Can you work these out from the model? Positions are in its coordinate system, mm. A direction names the side the tool comes from. Coordinates: 2 decimals unless noted, no trailing zeros. Order: outer loops, then holes, each group sorted by start corner. A loop starts at its lowest first (then second) coordinate and runs counter-clockwise, first axis right, second up. Notation, with made-up numbers: (-6.5, 77) -> (1.5, 77) arc R7 ccw to (1.5, 85) -> close; hole circle Ø1 at (50.5, 83). An arc over 180 degrees is marked (long way). Answer as a JSON object with one key per item and string values. Group by question number.
(1) For pin 1 (1.5 mm diameter, centred on x = -2.5, z = 3.5, fed in from -Y); pin 2 (2 mm diameter, centred on y = -2, z = 5.5, fed in from -X), each with a flat end and sliding along its axis, tell me the tip position at first contact or that it passes through.
(2) I want a section at A-A, the plane x = 6. List the corners of the cut face in (y, z) for me.
(3) I need wall thicknesses on line 1 (Y direction, x = 1, z = 5.5); line 2 (Y direction, x = 6.5, z = 1.25); line 3 (Y direction, x = -10.25, z = 2.5). Which ranges of each line are inside material? Lowest first, please.
(4) If we mould it in two halves opening along Y, with no side actions, what happens to faces 6 (the cylindrical face through (-12.62, -1.44, 3.13)), 7 (the cylindrical face through (12.62, 1.44, 3.13)), 8 (the cylindrical face through (7.67, -8.13, 3.13))? For each: pulls with the +Y half, pulls with the -Y half, needs draft (parallel to the pull), parting line crosses it, or undercut.
(5) I want a section at B-B, the plane z = 3. State how many separate pieces and enclosed holes the cut face has, plus the area to 3 significant figures.
(6) I want a section at C-C, the plane y = -4. List the corners of the cut face in (x, z) for me.
(7) Which directions (+Z, -Z, +X, -X, +Y, -Y) give clear straight access to the entire face, cutting with the end or side of a thin tool? Please do faces 1 (the cylindrical face through (-9.66, -5.51, 3.13)), 2 (the cylindrical face through (-2.44, 8.54, 3.13)), 3 (the cylindrical face through (5.51, -9.66, 3.13)), 4 (the cylindrical face through (7.895, 4.048, 3.131)), 5 (the cylindrical face through (-5.51, 9.66, 3.13)).
from build123d import *

# Parameters (mm, degrees)
SKETCH3_R         = 12.7
GEARBODY_DEPTH    = 6.35
TOOTHCUT_DEPTH    = 20.05
CIRPATTERN1_COUNT = 12
BOREDIA_R         = 2.5
BOREDIA_R_2       = 1.27
BORE_DEPTH        = 12700


with BuildPart() as part:
    # Sketch3 → gearBody (new body)
    with BuildSketch(Plane.XY):
        Circle(SKETCH3_R)
    extrude(amount=GEARBODY_DEPTH)

    # Sketch2 → toothCut (cut, through all)
    with BuildSketch(Plane.XY):
        with BuildLine():
            ThreePointArc((8.504981128, -1.619352377), (8.564111751, -1.270037802), (8.608901587, -0.918596522))
            ThreePointArc((8.608901587, -0.918596522), (8.867488023, -0.436790342), (9.388953743, -0.272237485))
            ThreePointArc((9.388953743, -0.272237485), (11.599176183, 0.135890641), (13.30511426, 1.599252209))
            ThreePointArc((13.30511426, 1.599252209), (13.255912686, -1.96582094), (12.268366453, -5.391739765))
            ThreePointArc((12.268366453, -5.391739765), (11.060534793, -3.49627294), (9.063879737, -2.464274691))
            ThreePointArc((9.063879737, -2.464274691), (8.61261217, -2.155467755), (8.504981128, -1.619352377))
        make_face()
    toothcut = extrude(amount=TOOTHCUT_DEPTH, mode=Mode.SUBTRACT)

    # CirPattern1: toothCut ×12 about axis
    cirpattern1_axis = Axis((0, 0, 0), (0, 0, 1))
    for i in range(1, CIRPATTERN1_COUNT):
        add(toothcut.rotate(cirpattern1_axis, i * 360 / CIRPATTERN1_COUNT), mode=Mode.SUBTRACT)

    # boreDia → bore (cut, symmetric)
    with BuildSketch(Plane.XY):
        Circle(BOREDIA_R)
        with Locations((0, 6.35)):
            Circle(BOREDIA_R_2)
        with Locations((6.35, 0)):
            Circle(BOREDIA_R_2)
        with Locations((-6.35, 0)):
            Circle(BOREDIA_R_2)
        with Locations((0, -6.35)):
            Circle(BOREDIA_R_2)
    extrude(amount=BORE_DEPTH, both=True, mode=Mode.SUBTRACT)


solid = part.part
Computed values:
{
 "1": {"pin 1": "stops at y = -10.77", "pin 2": "stops at x = -12.66"},
 "2": {"outline": "(-10.03, 0) -> (-1.22, 0) -> (-1.22, 6.35) -> (-10.03, 6.35) -> close; (1.22, 0) -> (6.39, 0) -> (6.39, 6.35) -> (1.22, 6.35) -> close"},
 "3": {"line 1": "y = -12.66 to -7.13, -5.57 to -2.29, 2.29 to 5.57, 7.13 to 8.6", "line 2": "y = -10.31 to -6.53, -5.73 to -1.26, 1.26 to 6.48", "line 3": "y = -7.5 to -6.37, -2.6 to 0.26, 2.91 to 5.69"},
 "4": {"face 6": "pulls with the -Y half", "face 7": "pulls with the +Y half", "face 8": "undercut"},
 "5": {"separate pieces": "1", "enclosed holes": "5", "area": "318 mm2"},
 "6": {"outline": "(-7.88, 0) -> (11.53, 0) -> (11.53, 6.35) -> (-7.88, 6.35) -> close"},
 "7": {"face 1": "+Z, -Z, -X", "face 2": "+Z, -Z", "face 3": "+Z, -Z, -Y", "face 4": "+Z, -Z, +X", "face 5": "+Z, -Z, +Y"}
}
